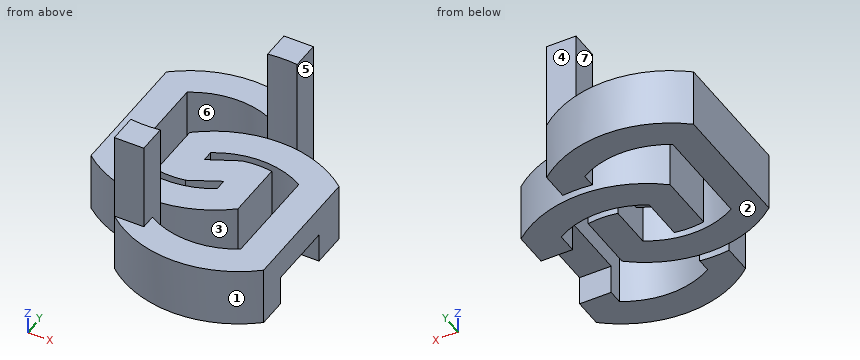
```python
from build123d import *

# Parameters (mm, degrees)
F1_DEPTH = 12.7
F2_DEPTH = 50.8
F0_W     = 13.666504261
F0_H     = 29.129663293
F3_DEPTH = 12.7


with BuildPart() as f1:
    # F0 (on Top) → F1 (new body)
    with BuildSketch(Plane.XY):
        with BuildLine():
            ThreePointArc((3.0578177724, 47.1438282191), (-28.6921822276, 58.6511969227), (-60.4421822276, 47.1438282191))
            Line((-60.4421822276, 47.1438282191), (-60.4421822276, -9.8514343737))
            ThreePointArc((-60.4421822276, -9.8514343737), (-28.6921822276, -21.3588030773), (3.0578177724, -9.8514343737))
            Line((3.0578177724, -9.8514343737), (3.0578177724, 15.7243934782))
            ThreePointArc((3.0578177724, 15.7243934782), (-3.3005283958, 16.2251409604), (-9.6421822276, 15.5448904828))
            Line((-9.6421822276, 15.5448904828), (-9.6421822276, 1.6402346703))
            Line((-9.6421822276, 1.6402346703), (-9.6421822276, -3.3534845781))
            ThreePointArc((-9.6421822276, -3.3534845781), (-28.6921822276, -8.6588030681), (-47.7421822276, -3.3534845781))
            Line((-47.7421822276, -3.3534845781), (-47.7421822276, 40.6458784342))
            ThreePointArc((-47.7421822276, 40.6458784342), (-28.6921822276, 45.9511969227), (-9.6421822276, 40.6458784342))
            Line((-9.6421822276, 40.6458784342), (-9.6421822276, 47.1438282191))
            Line((-9.6421822276, 47.1438282191), (3.0578177724, 47.1438282191))
        make_face()
        with BuildLine():
            Line((3.0578177724, 34.9553501383), (3.0578177724, 47.1438282191))
            Line((3.0578177724, 47.1438282191), (-9.6421822276, 47.1438282191))
            Line((-9.6421822276, 47.1438282191), (-9.6421822276, 40.6458784342))
            Line((-9.6421822276, 40.6458784342), (-9.6421822276, 34.8409533928))
            ThreePointArc((-9.6421822276, 34.8409533928), (-3.2955894398, 35.2764107322), (3.0578177724, 34.9553501383))
        make_face()
    extrude(amount=-F1_DEPTH)

    # F0 (on Top) → F2 (join)
    with BuildSketch(Plane.XY):
        with BuildLine():
            Line((3.0578177724, 34.9553501383), (3.0578177724, 47.1438282191))
            Line((3.0578177724, 47.1438282191), (-9.6421822276, 47.1438282191))
            Line((-9.6421822276, 47.1438282191), (-9.6421822276, 40.6458784342))
            Line((-9.6421822276, 40.6458784342), (-9.6421822276, 34.8409533928))
            ThreePointArc((-9.6421822276, 34.8409533928), (-3.2955894398, 35.2764107322), (3.0578177724, 34.9553501383))
        make_face()
    extrude(amount=F2_DEPTH)



with BuildPart() as f1b:
    # F0 (on Top) → F1, piece 2 (new body)
    with BuildSketch(Plane.XY):
        with BuildLine():
            Line((-22.3420616333, -4.8797410205), (-22.3420616333, 9.2116537254))
            Line((-22.3420616333, 9.2116537254), (-22.3420616333, 13.9284846169))
            ThreePointArc((-22.3420616333, 13.9284846169), (-3.2920616333, 19.2338031054), (15.7579383667, 13.9284846169))
            Line((15.7579383667, 13.9284846169), (15.7579383667, 5.2839141095))
            Line((15.7579383667, 5.2839141095), (29.4244426276, 5.2839141095))
            Line((29.4244426276, 5.2839141095), (29.4244426276, 20.4192625928))
            ThreePointArc((29.4244426276, 20.4192625928), (-2.8137786862, 32.1035806717), (-35.052, 20.4192625928))
            Line((-35.052, 20.4192625928), (-35.052, -4.8778777905))
            ThreePointArc((-35.052, -4.8778777905), (-28.6971195064, -5.4838027062), (-22.3420616333, -4.8797410205))
        make_face()
    extrude(amount=-F1_DEPTH)


with BuildPart() as f1c:
    # F0 (on Top) → F1, piece 3 (new body)
    with BuildSketch(Plane.XY):
        with BuildLine():
            Line((29.4244426276, -23.8457491835), (15.7579383667, -23.8457491835))
            Line((15.7579383667, -23.8457491835), (15.7579383667, -30.0708783954))
            ThreePointArc((15.7579383667, -30.0708783954), (-3.2920616333, -35.3761968854), (-22.3420616333, -30.0708783954))
            Line((-22.3420616333, -30.0708783954), (-22.3420616333, -36.576))
            Line((-22.3420616333, -36.576), (-35.052, -36.576))
            ThreePointArc((-35.052, -36.576), (-2.8137786862, -48.4961576662), (29.4244426276, -36.576))
            Line((29.4244426276, -36.576), (29.4244426276, -23.8457491835))
        make_face()
        with BuildLine():
            Line((-22.3420616333, -36.576), (-22.3420616333, -30.0708783954))
            Line((-22.3420616333, -30.0708783954), (-22.3420616333, -24.150039099))
            ThreePointArc((-22.3420616333, -24.150039099), (-28.6970664182, -24.5338028511), (-35.052, -24.1488618101))
            Line((-35.052, -24.1488618101), (-35.052, -24.150039099))
            Line((-35.052, -24.150039099), (-35.052, -36.576))
            Line((-35.052, -36.576), (-22.3420616333, -36.576))
        make_face()
    extrude(amount=-F1_DEPTH)

    # F0 (on Top) → F2, piece 2 (join)
    with BuildSketch(Plane.XY):
        with BuildLine():
            Line((-22.3420616333, -36.576), (-22.3420616333, -30.0708783954))
            Line((-22.3420616333, -30.0708783954), (-22.3420616333, -24.150039099))
            ThreePointArc((-22.3420616333, -24.150039099), (-28.6970664182, -24.5338028511), (-35.052, -24.1488618101))
            Line((-35.052, -24.1488618101), (-35.052, -24.150039099))
            Line((-35.052, -24.150039099), (-35.052, -36.576))
            Line((-35.052, -36.576), (-22.3420616333, -36.576))
        make_face()
    extrude(amount=F2_DEPTH)


with BuildPart() as f1_1:
    add(f1.part)

    add(f1b.part)  # F3 merges F1b

    add(f1c.part)  # F3 merges F1c
    # F0 (on Top) → F3 (join)
    with BuildSketch(Plane.XY):
        with BuildLine():
            ThreePointArc((3.0578177724, 47.1438282191), (-28.6921822276, 58.6511969227), (-60.4421822276, 47.1438282191))
            Line((-60.4421822276, 47.1438282191), (-60.4421822276, -9.8514343737))
            ThreePointArc((-60.4421822276, -9.8514343737), (-28.6921822276, -21.3588030773), (3.0578177724, -9.8514343737))
            Line((3.0578177724, -9.8514343737), (3.0578177724, 15.7243934782))
            ThreePointArc((3.0578177724, 15.7243934782), (-3.3005283958, 16.2251409604), (-9.6421822276, 15.5448904828))
            Line((-9.6421822276, 15.5448904828), (-9.6421822276, 1.6402346703))
            Line((-9.6421822276, 1.6402346703), (-9.6421822276, -3.3534845781))
            ThreePointArc((-9.6421822276, -3.3534845781), (-28.6921822276, -8.6588030681), (-47.7421822276, -3.3534845781))
            Line((-47.7421822276, -3.3534845781), (-47.7421822276, 40.6458784342))
            ThreePointArc((-47.7421822276, 40.6458784342), (-28.6921822276, 45.9511969227), (-9.6421822276, 40.6458784342))
            Line((-9.6421822276, 40.6458784342), (-9.6421822276, 47.1438282191))
            Line((-9.6421822276, 47.1438282191), (3.0578177724, 47.1438282191))
        make_face()
        with BuildLine():
            Line((-22.3420616333, -4.8797410205), (-22.3420616333, 9.2116537254))
            Line((-22.3420616333, 9.2116537254), (-22.3420616333, 13.9284846169))
            ThreePointArc((-22.3420616333, 13.9284846169), (-3.2920616333, 19.2338031054), (15.7579383667, 13.9284846169))
            Line((15.7579383667, 13.9284846169), (15.7579383667, 5.2839141095))
            Line((15.7579383667, 5.2839141095), (29.4244426276, 5.2839141095))
            Line((29.4244426276, 5.2839141095), (29.4244426276, 20.4192625928))
            ThreePointArc((29.4244426276, 20.4192625928), (-2.8137786862, 32.1035806717), (-35.052, 20.4192625928))
            Line((-35.052, 20.4192625928), (-35.052, -4.8778777905))
            ThreePointArc((-35.052, -4.8778777905), (-28.6971195064, -5.4838027062), (-22.3420616333, -4.8797410205))
        make_face()
        Polygon((-9.6421822276, 1.6402346703), (-9.6421822276, 15.5448904828), (-22.3420616333, 9.2116537254), (-22.3420616333, -4.8797410205), align=None)
        with Locations((22.5911904972, -9.280917537)):
            Rectangle(F0_W, F0_H)
        with BuildLine():
            Line((29.4244426276, -23.8457491835), (15.7579383667, -23.8457491835))
            Line((15.7579383667, -23.8457491835), (15.7579383667, -30.0708783954))
            ThreePointArc((15.7579383667, -30.0708783954), (-3.2920616333, -35.3761968854), (-22.3420616333, -30.0708783954))
            Line((-22.3420616333, -30.0708783954), (-22.3420616333, -36.576))
            Line((-22.3420616333, -36.576), (-35.052, -36.576))
            ThreePointArc((-35.052, -36.576), (-2.8137786862, -48.4961576662), (29.4244426276, -36.576))
            Line((29.4244426276, -36.576), (29.4244426276, -23.8457491835))
        make_face()
    extrude(amount=F3_DEPTH)


solid = f1_1.part
```
The listing builds one solid part. Answer for the finished solid, in the listing's coordinates (mm). Face numbers are marked on the shaded views. A direction names the side the tool comes from. Round coordinates to 2 decimals unless told otherwise and drop trailing zeros. Write each loop counter-clockwise with the first axis right and the second up, starting at its lowest first coordinate (ties: lowest second). Pieces come first, ordered by that corner, then holes. Notation, with made-up numbers: (-40, -33.75) -> (-16, -33.75) arc R14 ccw to (-16, -17.75) -> close; hole circle Ø11 at (40, -18.5). An arc over 180 degrees is marked (long way). Answer as a JSON object with one key per item and string values. Group by question number.
Q1. Which of the six approach directions +Z, -Z, +X, -X, +Y, -Y give full straight-line access (tool end or side, diameter ignored) to the marked faces 4, 5, 6 and 7?
Q2. Straight lines are drawn through the part: line 1 along Y through (x, z) = (-18.5, 10); line 2 along X through (y, z) = (37, 8); line 3 along X through (y, z) = (14.5, 12.5). For each, find the intervals that lie inside material, in ascending order.
Q3. Section A-A (z = -3.5) is taken. Write down the section's boundary in (x, y), plus the area to 3 significant figures.
Q4. Each of these flat-tipped pins is pushed along its axis until it touches: pin 1 Ø7 at (x, y) = (22, -9) entering from -Z; pin 2 Ø2 at (x, z) = (-8, 26.5) entering from -Y; pin 3 Ø4 at (x, z) = (19.5, -3.5) entering from -Y. Where does it stop, or does it pass through?
Q5. Section B-B (z = 14) is taken. Write down the section's boundary in (x, y), plus the area to 3 significant figures.
Q6. Determine the mould class of the marked faces 1, 2 and 3 for opening direction Y: pulls with the +Y half, pulls with the -Y half, needs draft (parallel to the pull), parting line crosses it, or undercut.
Q7. Section D-D (y = -32) is taken. Write down the section's boundary in (x, z), plus the area to 3 significant figures.
Q8. Section C-C (x = -19) is taken. Write down the section's boundary in (y, z).
Check values:
{
 "1": {"face 4": "+Z, +X, -X, +Y", "face 5": "+Z, -Z, +X, +Y", "face 6": "+Z, -Z", "face 7": "+Z"},
 "2": {"line 1": "-45.95 to -32.09, -20.3 to -7.22, -2.91 to 11.13, 15.95 to 29.6, 44.51 to 57.59", "line 2": "-60.44 to -47.74, -9.64 to 3.06", "line 3": "-60.44 to -47.74, -35.05 to -21.36, -11.74 to 3.06, 14.78 to 29.42"},
 "3": {"outline": "(-60.44, -9.85) arc R49.55 ccw to (3.06, -9.85) -> (3.06, 15.72) arc R34.44 ccw to (-9.64, 15.54) -> (-9.64, -3.35) arc R36.85 cw to (-47.74, -3.35) -> (-47.74, 40.65) arc R36.85 cw to (-9.64, 40.65) -> (-9.64, 34.84) arc R53.49 cw to (3.06, 34.96) -> (3.06, 47.14) arc R49.55 ccw to (-60.44, 47.14) -> close; (-35.05, -36.58) arc R49.55 ccw to (29.42, -36.58) -> (29.42, -23.85) -> (15.76, -23.85) -> (15.76, -30.07) arc R36.85 cw to (-22.34, -30.07) -> (-22.34, -24.15) arc R52.73 cw to (-35.05, -24.15) -> close; (-35.05, -4.88) arc R33.68 ccw to (-22.34, -4.88) -> (-22.34, 13.93) arc R36.85 cw to (15.76, 13.93) -> (15.76, 5.28) -> (29.42, 5.28) -> (29.42, 20.42) arc R50.32 ccw to (-35.05, 20.42) -> close", "area": "4,550 mm^2"},
 "4": {"pin 1": "z = 0", "pin 2": "y = 34.92", "pin 3": "y = -44.14"},
 "5": {"outline": "(-35.05, -36.58) -> (-22.34, -36.58) -> (-22.34, -24.15) arc R52.73 cw to (-35.05, -24.15) -> close; (-9.64, 34.84) arc R53.49 cw to (3.06, 34.96) -> (3.06, 47.14) -> (-9.64, 47.14) -> close", "area": "307 mm^2"},
 "6": {"face 1": "pulls with the -Y half", "face 2": "needs draft", "face 3": "undercut"},
 "7": {"outline": "(-35.05, -12.7) -> (-18.7, -12.7) -> (-18.7, 12.7) -> (-22.34, 12.7) -> (-22.34, 50.8) -> (-35.05, 50.8) -> close; (12.12, -12.7) -> (29.42, -12.7) -> (29.42, 12.7) -> (12.12, 12.7) -> close", "area": "1,340 mm^2"},
 "8": {"outline": "(-45.78, -12.7) -> (-31.86, -12.7) -> (-31.86, 12.7) -> (-45.78, 12.7) -> close; (-20.4, -12.7) -> (-7.36, -12.7) -> (-7.36, 12.7) -> (-20.4, 12.7) -> close; (-3.16, 0) -> (10.88, 0) -> (10.88, 12.7) -> (-3.16, 12.7) -> close; (15.72, -12.7) -> (29.43, -12.7) -> (29.43, 12.7) -> (15.72, 12.7) -> close; (44.65, -12.7) -> (57.69, -12.7) -> (57.69, 12.7) -> (44.65, 12.7) -> close"}
}
